from build123d import *

# Parameters (mm, degrees)
F1_DEPTH = 5.207
F2_R     = 10.16
F3_DEPTH = 5.207
F4_R     = 5.08


with BuildPart() as f1:
    # F0 (on Top) → F1 (new body)
    with BuildSketch(Plane.XY):
        Polygon((-44.776442, -50.8), (56.823558, -50.8), (56.823558, 10.39734), (-6.647165, 50.8), align=None)
    extrude(amount=F1_DEPTH)

    # F2 (on face) → F3 (cut, through all)
    with BuildSketch(Plane.XY.offset(5.207)):
        with Locations((33.963558, -15.907511)):
            Circle(F2_R)
    extrude(amount=-F3_DEPTH, mode=Mode.SUBTRACT)

    # F4
    f4_edges = [f1.edges().sort_by_distance(p)[0] for p in [
        (56.823558, -50.8, 2.6035),
        (-44.776442, -50.8, 2.6035),
    ]]
    fillet(f4_edges, radius=F4_R)


solid = f1.part
Could you check a few things on this model? Use its own coordinates, in mm. Coordinates: 2 decimals unless noted, no trailing zeros. Write each loop counter-clockwise with the first axis right and the second up, starting at its lowest first coordinate (ties: lowest second). Pieces come first, ordered by that corner, then holes. Notation, with made-up numbers: (-28, 36) - (-16, 36) arc R33 cw to (-16, 67) - close; hole circle Ø3 at (88, -5.5). An arc over 180 degrees is marked (long way). Put each result on its own line as item: value. Start each with the question number.
Q1. I want a section at B-B on z = 1.7. Write out the boundary of the cut face in (x, y).
Q2. I'm going to push a flat-ended pin straight in: P1, Ø1, axis at x = -4.5, z = 2.5, coming from the +Y side. Where does the tip first touch, or does it pass through?
Q3. Please list where these lines run through material, in increasing order: L1, parallel to X at y = -6.5, z = 3.8; L2, parallel to Y at x = 38, z = 3.95; L3, parallel to X at y = -19.5, z = 3.45.
Q4. I want a section at D-D on x = -36. Write out the boundary of the cut face in (y, z), plus the area to 3 significant figures.
Q5. I want a section at A-A on y = -21. Write out the boundary of the cut face in (x, z), plus the area to 3 significant figures.
Q6. Thinking about a two-plate mould opening in Y: for faces 1 (the cylindrical face through (55.3, -49.35, 2.64)), 2 (the cylindrical face through (25.9, -22.09, 2.64)), 3 (the flat face through (56.824, -18, 3)), which applies, pulls with the +Y half, pulls with the -Y half, needs draft (parallel to the pull), parting line crosses it, or undercut?
Q7. I want a section at C-C on x = 39. Write out the boundary of the cut face in (y, z), plus the area to 3 significant figures.
Checks:
1. outline: (-42.2, -43.94) arc R5.08 ccw to (-37.44, -50.8) - (51.74, -50.8) arc R5.08 ccw to (56.82, -45.72) - (56.82, 10.4) - (-6.65, 50.8) - close; hole circle Ø20.32 at (33.96, -15.91)
2. P1: y = 49.75
3. L1: -28.15 to 30.13, 37.8 to 56.82
3. L2: -50.8 to -25.23, -6.58 to 22.38
3. L3: -33.03 to 24.46, 43.47 to 56.82
4. outline: (-50.8, 0) - (-27.41, 0) - (-27.41, 5.21) - (-50.8, 5.21) - close
4. area: 122 mm²
5. outline: (-33.59, 0) - (25.17, 0) - (25.17, 5.21) - (-33.59, 5.21) - close; (42.76, 0) - (56.82, 0) - (56.82, 5.21) - (42.76, 5.21) - close
5. area: 379 mm²
6. face 1: pulls with the -Y half
6. face 2: undercut
6. face 3: needs draft
7. outline: (-50.8, 0) - (-24.73, 0) - (-24.73, 5.21) - (-50.8, 5.21) - close; (-7.08, 0) - (21.74, 0) - (21.74, 5.21) - (-7.08, 5.21) - close
7. area: 286 mm²
